from build123d import *

# Parameters (mm, degrees)
F1_DEPTH = 4.4
F3_DEPTH = 1.95
F6_R     = 1.475
F8_DEPTH = 2.6
F6_R_2   = 1.975
F9_DEPTH = 1
F10_R    = 1


# Not quite as in the source:
# - a pattern or mirror of a feature is missing from the dataset's text; its kind, count and spacing are read off the source's solid


with BuildPart() as f1:
    # F0 (on Top) → F1 (new body)
    with BuildSketch(Plane.XY):
        with BuildLine():
            Line((-60, 0), (0, 0))
            Line((0, 0), (0, 34))
            Line((0, 34), (-60, 34))
            ThreePointArc((-60, 34), (-62.8284271247, 32.8284271247), (-64, 30))
            Line((-64, 30), (-64, 4))
            ThreePointArc((-64, 4), (-62.8284271247, 1.1715728753), (-60, 0))
        make_face()
    extrude(amount=F1_DEPTH)

    # F2 (on face) → F3 (cut)
    with BuildSketch(Plane(origin=(0, 0, 0), x_dir=(1, 0, 0), z_dir=(0, 0, -1))):
        with BuildLine():
            ThreePointArc((-15.5, -34), (-16.9142135624, -33.4142135624), (-17.5, -32))
            Line((-17.5, -32), (-17.5, -30.5))
            ThreePointArc((-17.5, -30.5), (-16.9142135624, -29.0857864376), (-15.5, -28.5))
            Line((-15.5, -28.5), (-4, -28.5))
            Line((-4, -28.5), (-4, -5.5))
            Line((-4, -5.5), (-15.5, -5.5))
            ThreePointArc((-15.5, -5.5), (-16.9142135624, -4.9142135624), (-17.5, -3.5))
            Line((-17.5, -3.5), (-17.5, -2))
            ThreePointArc((-17.5, -2), (-16.9142135624, -0.5857864376), (-15.5, 0))
            Line((-15.5, 0), (-64, 0))
            Line((-64, 0), (-64, -34))
            Line((-64, -34), (-15.5, -34))
        make_face()
    extrude(amount=-F3_DEPTH, mode=Mode.SUBTRACT)

    # F6 (on face) → F8 (cut)
    with BuildSketch(Plane.XZ):
        with Locations((-2.4, 2.2)):
            Circle(F6_R)
    f8 = extrude(amount=-F8_DEPTH, mode=Mode.SUBTRACT)

    # F8_copies: F8 across plane
    add(f8.mirror(Plane.ZX.offset(17)), mode=Mode.SUBTRACT)

    # F6 (on face) → F9 (cut)
    with BuildSketch(Plane.XZ):
        with Locations((-2.4, 2.2)):
            Circle(F6_R_2)
        with Locations((-2.4, 2.2)):
            Circle(F6_R, mode=Mode.SUBTRACT)
    f9 = extrude(amount=-F9_DEPTH, mode=Mode.SUBTRACT)

    # F9_copies: F9 across plane
    add(f9.mirror(Plane.ZX.offset(17)), mode=Mode.SUBTRACT)

    # F10
    f10_edges = [f1.edges().sort_by_distance(p)[0] for p in [
        (0, 17, 4.4),
        (0, 17, 0),
    ]]
    fillet(f10_edges, radius=F10_R)


solid = f1.part
Design review of the part built by this model. Coordinates are the model's own, in mm. A direction names the side the tool comes from. Round coordinates to 2 decimals unless told otherwise and drop trailing zeros. Order: outer loops, then holes, each group sorted by start corner. A loop starts at its lowest first (then second) coordinate and runs counter-clockwise, first axis right, second up.
1) Consider section C-C (x = -33). State the section outline as (y, z) points.
The answers:
outline: (0, 1.95) - (34, 1.95) - (34, 4.4) - (0, 4.4) - close
2) Consider section B-B (x = -5). State the section outline as (y, z) points.
The answers:
outline: (0, 0) - (5.5, 0) - (5.5, 1.95) - (28.5, 1.95) - (28.5, 0) - (34, 0) - (34, 4.4) - (0, 4.4) - close
3) Clearance check with flat-ended pins moving along their axes: pin 1 Ø1.5 at (x, z) = (-2.5, 2) entering from -Y; pin 2 Ø2 at (x, z) = (-3.5, 2) entering from -Y; pin 3 Ø1 at (y, z) = (11.5, 1) entering from -X; pin 4 Ø2.5 at (x, z) = (-2, 2.5) entering from +Y. State where each tip first meets the part, or that it passes through.
The answers:
pin 1: stops at y = 2.6
pin 2: stops at y = 0
pin 3: stops at x = -4
pin 4: stops at y = 33
4) Draft analysis for pull direction Z (two halves, no side actions). For faces 1 (the flat face through (-34, 17, 1.95)), 2 (the cylindrical face through (-2.657, 33.507, 4.158)), 3 (the cylindrical face through (-16.9, 4.93, 0.96)), state which applies: released by +Z, released by -Z, zero draft, split by the parting line, or undercut.
The answers:
face 1: released by -Z
face 2: undercut
face 3: zero draft
5) For L1, parallel to Z at x = -2.4, y = 0.7 (3 decimals); L2, parallel to Y at x = -15, z = 0.6; L3, parallel to Z at x = -2.4, y = 32.45 (3 decimals), list the stretches that pass through material, from the lowest coordinate up.
The answers:
L1: z = 0 to 0.225, 4.175 to 4.4
L2: y = 0 to 5.5, 28.5 to 34
L3: z = 0 to 0.725, 3.675 to 4.4
6) Consider section A-A (y = 9.5). State the section outline as (x, z) points, plus the area to 3 significant figures.
The answers:
outline: (-64, 1.95) - (-4, 1.95) - (-4, 0) - (-1, 0) arc R1 ccw to (0, 1) - (0, 3.4) arc R1 ccw to (-1, 4.4) - (-64, 4.4) - close
area: 164 mm2
7) Machinability: for faces 4 (the flat face through (-2, 2.6, 2)), 5 (the cylindrical face through (-2.72, 32.21, 0.76)), 6 (the cylindrical face through (-16.93, 29.1, 0.96)), which of the approach directions +Z, -Z, +X, -X, +Y, -Y give a long, thin tool a straight path to every point of the face, cutting with its end or side? Answer none if there is none.
The answers:
face 4: -Y
face 5: +Y
face 6: -Z, -X
